from build123d import *

# Parameters (mm, degrees)
SKETCH1_W           = 19
SKETCH1_H           = 19
BOSS_EXTRUDE1_DEPTH = 20
SKETCH2_R           = 6.5
BOSS_EXTRUDE2_DEPTH = 2
SKETCH3_R           = 6.5
BOSS_EXTRUDE3_DEPTH = 13
BOSS_EXTRUDE4_DEPTH = 35
SKETCH5_R           = 11.75
BOSS_EXTRUDE5_DEPTH = 11


with BuildPart() as part:
    # Sketch1 → Boss-Extrude1 (new body)
    with BuildSketch(Plane.XY):
        with Locations((5.167364017, -0.218619247)):
            Rectangle(SKETCH1_W, SKETCH1_H)
    extrude(amount=BOSS_EXTRUDE1_DEPTH)

    # Sketch2 → Boss-Extrude2 (add)
    with BuildSketch(Plane.XY.offset(20)):
        with Locations((5.218963732, -0.412118181)):
            Circle(SKETCH2_R)
    extrude(amount=BOSS_EXTRUDE2_DEPTH)

    # Sketch3 → Boss-Extrude3 (add)
    with BuildSketch(Plane(origin=(0, 0, 0), x_dir=(-1, 0, 0), z_dir=(0, 0, -1))):
        with Locations((-5.167364017, -0.218619247)):
            Circle(SKETCH3_R)
    extrude(amount=BOSS_EXTRUDE3_DEPTH)

    # Sketch4 → Boss-Extrude4 (add)
    with BuildSketch(Plane(origin=(0, 9.281380753, 0), x_dir=(1, 0, 0), z_dir=(0, 1, 0))):
        Polygon((14.404968324, -10), (9.78616617, -2), (0.548561863, -2), (-4.07024029, -10), (0.548561863, -18), (9.78616617, -18), align=None)
    extrude(amount=BOSS_EXTRUDE4_DEPTH)

    # Sketch5 → Boss-Extrude5 (add)
    with BuildSketch(Plane(origin=(0, 44.281380753, 0), x_dir=(1, 0, 0), z_dir=(0, 1, 0))):
        with Locations((5.167364017, -10)):
            Circle(SKETCH5_R)
    extrude(amount=-BOSS_EXTRUDE5_DEPTH)


solid = part.part
Design review of the part built by this model. Coordinates are the model's own, in mm. A direction names the side the tool comes from. Coordinates: 2 decimals unless noted, no trailing zeros. Loops run counter-clockwise (first coordinate to the right, second up) from the corner with the lowest first, then second, coordinate; pieces in that order, holes last. Notation, with made-up numbers: M 65.25,80.5 L 118.25,80.5 A21 ccw 118.25,101.5 Z; hole C 67,-26.5 d4. An arc over 180 degrees is marked long. Answer as CSV lines item,"result".
Item 1: The part is to be moulded in two halves that separate along Y. For faces 1 (the face through (14.667, 0, 10)), 2 (the face through (5, -9.719, 10)), 3 (the face through (5.03, 6.25, 20)), say which applies: pulls with the +Y half, pulls with the -Y half, needs draft (parallel to the pull), parting line crosses it, or undercut.
Answer list:
face 1,"needs draft"
face 2,"pulls with the -Y half"
face 3,"undercut"
Item 2: Add section A-A on y = 22. State the section outline as (x, z) points, plus the area to 3 significant figures.
Answer list:
outline,"M -4.07,10 L 0.55,2 L 9.79,2 L 14.4,10 L 9.79,18 L 0.55,18 Z"
area,"222 mm²"
Item 3: Machinability: for faces 4 (the face through (5, 21, 18)), 5 (the face through (-3.4, 9.281, 7.6)), 6 (the face through (11.66, 0.07, -6.41)), 7 (the face through (-1.729, 21.113, 5.944)), 8 (the face through (5, 21, 2)), which of the approach directions +Z, -Z, +X, -X, +Y, -Y give a long, thin tool a straight path to every point of the face, cutting with its end or side? Answer none if there is none.
Answer list:
face 4,"+Z, +X, -X"
face 5,"none"
face 6,"-Z"
face 7,"-Z, -X"
face 8,"-Z, +X, -X"
Item 4: For P1, Ø9.5, axis at y = -4.5, z = 5.5, coming from the -X side; P2, Ø8, axis at x = 4.5, y = 37, coming from the +Z side; P3, Ø7.5, axis at x = 7, y = 19, coming from the -Z side, all flat-tipped, find the tip position at first contact; note any pin that passes through.
Answer list:
P1,"x = -4.33"
P2,"z = 21.75"
P3,"z = 2"
Item 5: Add section D-D on x = -2.5. State the section outline as (y, z) points.
Answer list:
outline,"M -9.72,0 L 9.28,0 L 9.28,7.28 L 33.28,7.28 L 33.28,1.1 L 44.28,1.1 L 44.28,18.9 L 33.28,18.9 L 33.28,12.72 L 9.28,12.72 L 9.28,20 L -9.72,20 Z"
Item 6: Add section B-B on z = 16.5. State the section outline as (x, y) points, plus the area to 3 significant figures.
Answer list:
outline,"M -4.62,33.28 L -0.32,33.28 L -0.32,9.28 L -4.33,9.28 L -4.33,-9.72 L 14.67,-9.72 L 14.67,9.28 L 10.65,9.28 L 10.65,33.28 L 14.96,33.28 L 14.96,44.28 L -4.62,44.28 Z"
area,"840 mm²"
Item 7: Add section C-C on x = 5. State the section outline as (y, z) points, plus the area to 3 significant figures.
Answer list:
outline,"M -9.72,0 L -6.72,0 L -6.72,-13 L 6.28,-13 L 6.28,0 L 9.28,0 L 9.28,2 L 33.28,2 L 33.28,-1.75 L 44.28,-1.75 L 44.28,21.75 L 33.28,21.75 L 33.28,18 L 9.28,18 L 9.28,20 L 6.08,20 L 6.08,22 L -6.91,22 L -6.91,20 L -9.72,20 Z"
area,"1,220 mm²"
Item 8: For probe 1 along Y at (x, z) = (7.75, 0.5); probe 2 along Z at (x, y) = (7, 29.5); probe 3 along X at (y, z) = (6, 12), list the stretches that pass through material, from the lowest coordinate up.
Answer list:
probe 1,"-9.72 to 9.28, 33.28 to 44.28"
probe 2,"2 to 18"
probe 3,"-4.33 to 14.67"
